Check sheet for the modelled part. Datum: model origin and axes. Units: mm. A direction names the side the tool comes from. Give positions to 0.01 mm unless a question says otherwise; leave off trailing zeros. Order: outer loops, then holes, each group sorted by start corner. A loop starts at its lowest first (then second) coordinate and runs counter-clockwise, first axis right, second up.
from build123d import *

# Parameters (mm, degrees)
BOSS_EXTRUDE1_DEPTH = 10
SKETCH3_W           = 17.2
SKETCH3_H           = 43
CUT_EXTRUDE1_DEPTH  = 72.414284285
SKETCH5_W           = 49.6
SKETCH5_H           = 5
BOSS_EXTRUDE3_DEPTH = 12
BOSS_EXTRUDE2_START = -12
SKETCH2_W           = 34
SKETCH2_H           = 90
SKETCH2_W_2         = 24
SKETCH2_H_2         = 80
BOSS_EXTRUDE2_DEPTH = 27
SKETCH6_W           = 5
SKETCH6_H           = 10
CUT_EXTRUDE2_DEPTH  = 27
SKETCH8_W           = 24
SKETCH8_H           = 48.5
SKETCH8_H_2         = 11.5
BOSS_EXTRUDE4_DEPTH = 12


with BuildPart() as part:
    # Sketch1 → Boss-Extrude1 (new body)
    with BuildSketch(Plane(origin=(0, 0, 0), x_dir=(1, 0, 0), z_dir=(0, 1, 0))):
        with BuildLine():
            Line((-35, 50), (35, 50))
            ThreePointArc((35, 50), (45.606601718, 45.606601718), (50, 35))
            Line((50, 35), (50, -35))
            ThreePointArc((50, -35), (45.606601718, -45.606601718), (35, -50))
            Line((35, -50), (-35, -50))
            ThreePointArc((-35, -50), (-45.606601718, -45.606601718), (-50, -35))
            Line((-50, -35), (-50, 35))
            ThreePointArc((-50, 35), (-45.606601718, 45.606601718), (-35, 50))
        make_face()
    extrude(amount=BOSS_EXTRUDE1_DEPTH)

    # Sketch3 → Cut-Extrude1 (cut, through all)
    with BuildSketch(Plane(origin=(0, 10, 0), x_dir=(1, 0, 0), z_dir=(0, 1, 0))):
        with Locations((-33.4, 18.5)):
            Rectangle(SKETCH3_W, SKETCH3_H)
        with Locations((33.4, 18.5)):
            Rectangle(SKETCH3_W, SKETCH3_H)
    extrude(amount=-CUT_EXTRUDE1_DEPTH, mode=Mode.SUBTRACT)

    # Sketch5 → Boss-Extrude3 (add)
    with BuildSketch(Plane(origin=(0, 10, 0), x_dir=(1, 0, 0), z_dir=(0, 1, 0))):
        with Locations((0, 11)):
            Rectangle(SKETCH5_W, SKETCH5_H)
        with Locations((0, 26)):
            Rectangle(SKETCH5_W, SKETCH5_H)
    extrude(amount=BOSS_EXTRUDE3_DEPTH)

    # Sketch2 → Boss-Extrude2 (add)
    with BuildSketch(Plane(origin=(0, 22, 0), x_dir=(1, 0, 0), z_dir=(0, 1, 0)).offset(BOSS_EXTRUDE2_START)):
        Rectangle(SKETCH2_W, SKETCH2_H)
        Rectangle(SKETCH2_W_2, SKETCH2_H_2, mode=Mode.SUBTRACT)
    extrude(amount=BOSS_EXTRUDE2_DEPTH)

    # Sketch6 → Cut-Extrude2 (cut)
    with BuildSketch(Plane(origin=(0, 37, 0), x_dir=(1, 0, 0), z_dir=(0, 1, 0))):
        with Locations((-14.5, 18.5)):
            Rectangle(SKETCH6_W, SKETCH6_H)
        with Locations((14.5, 18.5)):
            Rectangle(SKETCH6_W, SKETCH6_H)
    extrude(amount=-CUT_EXTRUDE2_DEPTH, mode=Mode.SUBTRACT)

    # Sketch8 → Boss-Extrude4 (add)
    with BuildSketch(Plane(origin=(0, 10, 0), x_dir=(1, 0, 0), z_dir=(0, 1, 0))):
        with Locations((0, -15.75)):
            Rectangle(SKETCH8_W, SKETCH8_H)
        with Locations((0, 34.25)):
            Rectangle(SKETCH8_W, SKETCH8_H_2)
    extrude(amount=BOSS_EXTRUDE4_DEPTH)


solid = part.part
1) Draft check along Z on faces 1 (the face through (0, 23, -45)), 2 (the face through (0, 29, -40)), 3 (the face through (23, 10, -1)). Enter one of: +Z half, -Z half, draft (parallel to the pull), parting line (faces both ways), or undercut.
Recorded:
face 1: -Z half
face 2: undercut
face 3: draft
2) Section check C-C, the plane x = -27. Record the cut outline in (y, z).
Recorded:
outline: (0, -50) - (10, -50) - (10, -40) - (0, -40) - close; (0, 3) - (10, 3) - (10, 50) - (0, 50) - close
3) Section check B-B, the plane z = 1. Record the cut outline in (x, y).
Recorded:
outline: (-50, 0) - (-42, 0) - (-42, 10) - (-50, 10) - close; (-24.8, 0) - (24.8, 0) - (24.8, 10) - (17, 10) - (17, 37) - (12, 37) - (12, 22) - (-12, 22) - (-12, 37) - (-17, 37) - (-17, 10) - (-24.8, 10) - close; (42, 0) - (50, 0) - (50, 10) - (42, 10) - close
4) Depth check by flat-ended pin: pin 1 Ø5.5 at (x, z) = (-19.5, -10.5) entering from +Y; pin 2 Ø8 at (y, z) = (26.5, 22) entering from -X; pin 3 Ø1.5 at (x, y) = (4, 29) entering from -Z; pin 4 Ø4 at (x, y) = (3.5, 12.5) entering from +Z. Enter the tip coordinate at first touch or a pass-through.
Recorded:
pin 1: stops at y = 37
pin 2: stops at x = -17
pin 3: stops at z = -45
pin 4: stops at z = 45
5) Set-up check for faces 4 (the face through (0, 5, 50)), 5 (the face through (45.49, 4.93, -45.72)), 6 (the face through (42, 5, -18)), 7 (the face through (0, 23, 45)), 8 (the face through (-12, 29, -32)): record each of +Z, -Z, +X, -X, +Y, -Y from which the full face is reachable in a straight line by a thin tool's end or side.
Recorded:
face 4: +Z, +X, -X, +Y, -Y
face 5: -Z, +X, +Y, -Y
face 6: +Y, -Y
face 7: +Z, +X, -X, +Y
face 8: +Y
6) Section check D-D, the plane x = -6.5. Record the cut outline in (y, z).
Recorded:
outline: (0, -50) - (10, -50) - (10, -45) - (37, -45) - (37, -40) - (22, -40) - (22, -23.5) - (10, -23.5) - (10, -13.5) - (22, -13.5) - (22, 40) - (37, 40) - (37, 45) - (10, 45) - (10, 50) - (0, 50) - close
7) Material ranges on L1, parallel to X at y = 5.5, z = -26.5; L2, parallel to Z at x = 4, y = 26; L3, parallel to Z at x = -34.5, y = 2.5, recorded low to high.
Recorded:
L1: x = -50 to -42, -24.8 to 24.8, 42 to 50
L2: z = -45 to -40, 40 to 45
L3: z = -50 to -40, 3 to 50
8) Section check A-A, the plane y = 17. Record the cut outline in (x, z), then the cut area to 3 significant figures.
Recorded:
outline: (-24.8, -28.5) - (-17, -28.5) - (-17, -45) - (17, -45) - (17, -28.5) - (24.8, -28.5) - (24.8, -23.5) - (-24.8, -23.5) - close; (-24.8, -13.5) - (24.8, -13.5) - (24.8, -8.5) - (17, -8.5) - (17, 45) - (-17, 45) - (-17, -8.5) - (-24.8, -8.5) - close
area: 2,880 mm2
